Read the model definition and answer for the solid it produces. Units are mm, in the model's axes. A direction names the side the tool comes from. Coordinates: 2 decimals unless noted, no trailing zeros. Write each loop counter-clockwise with the first axis right and the second up, starting at its lowest first coordinate (ties: lowest second). Pieces come first, ordered by that corner, then holes. Notation, with made-up numbers: (77, -34) -> (133, -34) arc R24 ccw to (133, 3) -> close; hole circle Ø8 at (-8, 33.25). An arc over 180 degrees is marked (long way). Answer in a Markdown table with one row per item. Add a question column.
Item 1: For a pull along Y with two mould halves and no side action, classify faces 4 (the face through (-21.17, -24.57, 2.46)), 5 (the face through (0, 28.57, 2)), 6 (the face through (10.37, -38.75, 2.54)), 7 (the face through (7, -44, -13)) as +Y half, -Y half, draft (parallel to the pull), parting line (faces both ways), or undercut.
Item 2: Straight lines are drawn through the part: line 1 (Y direction, x = -23.57, z = 1.4); line 2 (Y direction, x = -23, z = 2); line 3 (Y direction, x = 0, z = 1). For each, find the intervals that lie inside material, in ascending order. Write a range as from..to.
Item 3: Section D-D on x = -8 is taken. Write down the section's boundary in (y, z).
Item 4: Which of the six approach directions +Z, -Z, +X, -X, +Y, -Y give full straight-line access (tool end or side, diameter ignored) to faces 1 (the face through (0, -52, -34.9)), 2 (the face through (-7, -44, -13)), 3 (the face through (20.13, -28.96, 2.54))?
Item 5: Section B-B on y = 0 is taken. Write down the section's boundary in (x, z).
Item 6: Section C-C on z = -22.5 is taken. Write down the section's boundary in (x, y), then the cut area to 3 significant figures.
Item 7: Section A-A on x = 0 is taken. Write down the section's boundary in (y, z), then the cut area to 3 significant figures.
Item 8: Given pin 1 Ø3 at (x, y) = (-23.57, 23.57) entering from -Z; pin 2 Ø17 at (x, y) = (-5.5, -15) entering from -Z; pin 3 Ø15.5 at (y, z) = (-37.5, -15) entering from -X; pin 4 Ø21.5 at (y, z) = (-36.5, -15) entering from +X, each flat-ended and moving along its own axis, determine where each tip first touches the part or whether it passes through.
```python
from build123d import *

# Parameters (mm, degrees)
SKETCH1_W           = 57.14
SKETCH1_H           = 57.14
SKETCH1_R           = 19.5
SKETCH1_R_2         = 2.6
SKETCH1_W_2         = 20
SKETCH1_H_2         = 26.43
BOSS_EXTRUDE1_DEPTH = 5
SKETCH3_W           = 45
SKETCH3_H           = 5
BOSS_EXTRUDE2_DEPTH = 20
BOSS_EXTRUDE3_START = -7.5
BOSS_EXTRUDE3_DEPTH = 5
CUT_EXTRUDE1_REACH  = 96.945
FILLET1_R           = 5
CHAMFER1_SIZE       = 4
CHAMFER2_SIZE       = 10
FILLET2_R           = 5
BOSS_EXTRUDE4_DEPTH = 3


with BuildPart() as part:
    # Sketch1 → Boss-Extrude1 (new body)
    # profile 1 of 2: a face of its own
    with BuildSketch(Plane.XY):
        Rectangle(SKETCH1_W, SKETCH1_H)
        Circle(SKETCH1_R, mode=Mode.SUBTRACT)
        with Locations((-23.57, -23.57)):
            Circle(SKETCH1_R_2, mode=Mode.SUBTRACT)
        with Locations((23.57, -23.57)):
            Circle(SKETCH1_R_2, mode=Mode.SUBTRACT)
        with Locations((23.57, 23.57)):
            Circle(SKETCH1_R_2, mode=Mode.SUBTRACT)
        with Locations((-23.57, 23.57)):
            Circle(SKETCH1_R_2, mode=Mode.SUBTRACT)
    # profile 2 of 2: a face of its own
    with BuildSketch(Plane.XY):
        with Locations((0, -41.785)):
            Rectangle(SKETCH1_W_2, SKETCH1_H_2)
    extrude(amount=BOSS_EXTRUDE1_DEPTH)

    # Sketch3 → Boss-Extrude2 (add)
    with BuildSketch(Plane(origin=(10, 0, 0), x_dir=(0, 0, -1), z_dir=(1, 0, 0))):
        with Locations((22.5, -52.5)):
            Rectangle(SKETCH3_W, SKETCH3_H)
    extrude(amount=-BOSS_EXTRUDE2_DEPTH)

    # Sketch5 → Boss-Extrude3 (add)
    with BuildSketch(Plane(origin=(10, 0, 0), x_dir=(0, 0, -1), z_dir=(1, 0, 0)).offset(BOSS_EXTRUDE3_START)):
        Polygon((0, -35), (15, -50), (0, -50), align=None)
    extrude(amount=-BOSS_EXTRUDE3_DEPTH)

    # Sketch4 → Cut-Extrude1 (cut, up to next)
    with BuildSketch(Plane(origin=(0, -50, 0), x_dir=(1, 0, 0), z_dir=(0, 1, 0)), mode=Mode.PRIVATE) as cut_extrude1_sk1:
        with BuildLine():
            Line((-2.5, 40.1), (2.5, 40.1))
            ThreePointArc((2.5, 40.1), (5.1, 37.5), (2.5, 34.9))
            Line((2.5, 34.9), (-2.5, 34.9))
            ThreePointArc((-2.5, 34.9), (-5.1, 37.5), (-2.5, 40.1))
        make_face()
    cut_extrude1_tool1 = extrude(cut_extrude1_sk1.sketch, amount=-CUT_EXTRUDE1_REACH, mode=Mode.PRIVATE) & part.part
    # Sketch4 → Cut-Extrude1 (cut, up to next)
    with BuildSketch(Plane(origin=(0, -50, 0), x_dir=(1, 0, 0), z_dir=(0, 1, 0)), mode=Mode.PRIVATE) as cut_extrude1_sk2:
        with BuildLine():
            Line((-2.5, 25.1), (2.5, 25.1))
            ThreePointArc((2.5, 25.1), (5.1, 22.5), (2.5, 19.9))
            Line((2.5, 19.9), (-2.5, 19.9))
            ThreePointArc((-2.5, 19.9), (-5.1, 22.5), (-2.5, 25.1))
        make_face()
    cut_extrude1_tool2 = extrude(cut_extrude1_sk2.sketch, amount=-CUT_EXTRUDE1_REACH, mode=Mode.PRIVATE) & part.part
    add(cut_extrude1_tool1.solids().sort_by_distance((0, -50, -37.5))[0], mode=Mode.SUBTRACT)
    add(cut_extrude1_tool2.solids().sort_by_distance((0, -50, -22.5))[0], mode=Mode.SUBTRACT)

    # Fillet1
    fillet1_edges = [part.edges().sort_by_distance(p)[0] for p in [
        (28.57, -28.57, 2.5),
        (-28.57, -28.57, 2.5),
        (-28.57, 28.57, 2.5),
        (28.57, 28.57, 2.5),
    ]]
    fillet(fillet1_edges, radius=FILLET1_R)

    # Chamfer1
    chamfer1_edges = [part.edges().sort_by_distance(p)[0] for p in [
        (-6.25, -50, 0),
        (6.25, -50, 0),
    ]]
    chamfer(chamfer1_edges, length=CHAMFER1_SIZE)

    # Chamfer2
    chamfer2_edges = [part.edges().sort_by_distance(p)[0] for p in [
        (10, -28.57, 2.5),
        (-10, -28.57, 2.5),
    ]]
    chamfer(chamfer2_edges, length=CHAMFER2_SIZE)

    # Fillet2
    fillet2_edges = [part.edges().sort_by_distance(p)[0] for p in [
        (-10, -38.57, 2.5),
        (-20, -28.57, 2.5),
        (20, -28.57, 2.5),
        (10, -38.57, 2.5),
    ]]
    fillet(fillet2_edges, radius=FILLET2_R)

    # Sketch6 → Boss-Extrude4 (add)
    with BuildSketch(Plane(origin=(10, 0, 0), x_dir=(0, 0, -1), z_dir=(1, 0, 0))):
        Polygon((45, -50), (4, -50), (0, -46), (0, -30.534466094), align=None)
    boss_extrude4 = extrude(amount=-BOSS_EXTRUDE4_DEPTH)

    # Mirror1: Boss-Extrude4 across plane
    add(boss_extrude4.mirror(Plane(origin=(0, 0, 0), x_dir=(0, 0, 1), z_dir=(1, 0, 0))))


solid = part.part
```
Results below:
| question | item | result |
|---|---|---|
| 1 | face 4 | undercut |
| 1 | face 5 | +Y half |
| 1 | face 6 | -Y half |
| 1 | face 7 | draft |
| 2 | line 1 | y = -28.57..-26.17, -20.97..20.97, 26.17..28.57 |
| 2 | line 2 | y = -28.57..-26.11, -21.03..21.03, 26.11..28.57 |
| 2 | line 3 | y = -55..-19.5, 19.5..28.57 |
| 3 | outline | (-55, -45) -> (-50, -45) -> (-30.53, 0) -> (-17.78, 0) -> (-17.78, 5) -> (-55, 5) -> close; (17.78, 0) -> (28.57, 0) -> (28.57, 5) -> (17.78, 5) -> close |
| 4 | face 1 | +Y, -Y |
| 4 | face 2 | -Z, +Y |
| 4 | face 3 | +Z, -Z, +X, -Y |
| 5 | outline | (-28.57, 0) -> (-19.5, 0) -> (-19.5, 5) -> (-28.57, 5) -> close; (19.5, 0) -> (28.57, 0) -> (28.57, 5) -> (19.5, 5) -> close |
| 6 | outline | (-10, -55) -> (-5.1, -55) -> (-5.1, -50) -> (-7, -50) -> (-7, -40.27) -> (-10, -40.27) -> close; (5.1, -55) -> (10, -55) -> (10, -40.27) -> (7, -40.27) -> (7, -50) -> (5.1, -50) -> close |
| 6 | area | 107 mm2 |
| 7 | outline | (-55, -45) -> (-50, -45) -> (-50, -40.1) -> (-55, -40.1) -> close; (-55, -34.9) -> (-50, -34.9) -> (-50, -25.1) -> (-55, -25.1) -> close; (-55, -19.9) -> (-50, -19.9) -> (-50, -15) -> (-35, 0) -> (-19.5, 0) -> (-19.5, 5) -> (-55, 5) -> close; (19.5, 0) -> (28.57, 0) -> (28.57, 5) -> (19.5, 5) -> close |
| 7 | area | 508 mm2 |
| 8 | pin 1 | passes through |
| 8 | pin 2 | stops at z = 0 |
| 8 | pin 3 | stops at x = -10 |
| 8 | pin 4 | stops at x = 10 |
